Can you work these out from the drawing? Everything is in mm from the part's minimum corner. A direction names the side the tool comes from. Coordinates: 2 decimals unless noted, no trailing zeros. Order: outer loops, then holes, each group sorted by start corner. A loop starts at its lowest first (then second) coordinate and runs counter-clockwise, first axis right, second up. Notation, with made-up numbers: (37.25, -20) -> (68.25, -20) arc R18 cw to (68.25, -5) -> close; hole circle Ø9 at (17.25, 47.25). An arc over 180 degrees is marked (long way). Put each result on its own line as item: value. Start each with the question number.
Q1. Please list where these lines run through material, in increasing order: line 1 along Y through (x, z) = (4.15, 5); line 2 along Z through (x, y) = (2.2, 17.75); line 3 along Z through (x, y) = (0.5, 10).
Q2. If we section it at B-B (x = 3): Please give me the cut outline in (y, z).
Q3. If we section it at A-A (y = 3): Please give me the cut outline in (x, z).
Q4. If we section it at D-D (y = 10.25): Please give me the cut outline in (x, z).
Q5. Will these pins go through, and if not, where does the flat tip stop? pin 1 (3 mm diameter, centred on x = 2, y = 21, fed in from -Z); pin 2 (1.9 mm diameter, centred on x = 3, y = 22.5, fed in from -Z); pin 3 (1 mm diameter, centred on x = 3, y = 12.5, fed in from -Z).
Q6. If we section it at C-C (z = 13.25): Please give me the cut outline in (x, y).
Q7. For the marked faces 1, 2 and 3, which set-ups out of +Z, -Z, +X, -X, +Y, -Y let a thin tool reach every point of the face, with its end or its side?
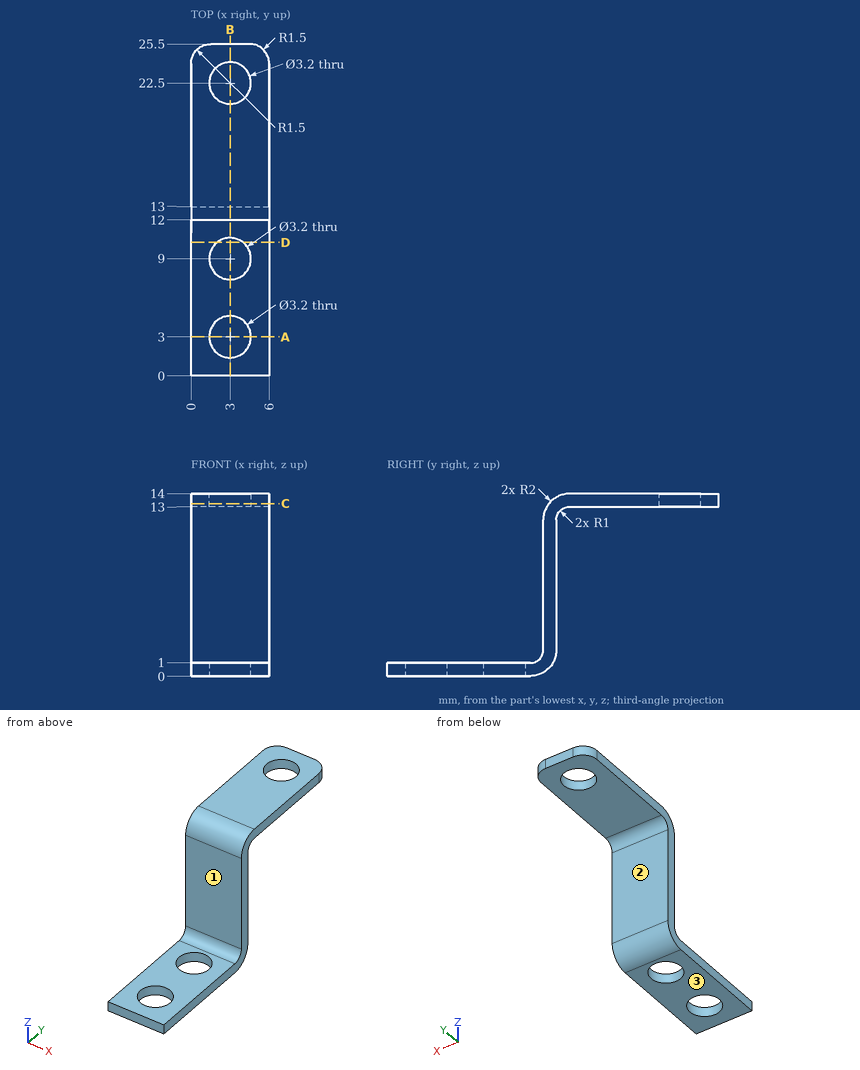
The answers:
1. line 1: 12 to 13
1. line 2: 13 to 14
1. line 3: 0 to 1
2. outline: (0, 0) -> (1.4, 0) -> (1.4, 1) -> (0, 1) -> close; (4.6, 0) -> (7.4, 0) -> (7.4, 1) -> (4.6, 1) -> close; (10.6, 0) -> (11, 0) arc R2 ccw to (13, 2) -> (13, 12) arc R1 cw to (14, 13) -> (20.9, 13) -> (20.9, 14) -> (14, 14) arc R2 ccw to (12, 12) -> (12, 2) arc R1 cw to (11, 1) -> (10.6, 1) -> close; (24.1, 13) -> (25.5, 13) -> (25.5, 14) -> (24.1, 14) -> close
3. outline: (0, 0) -> (1.4, 0) -> (1.4, 1) -> (0, 1) -> close; (4.6, 0) -> (6, 0) -> (6, 1) -> (4.6, 1) -> close
4. outline: (0, 0) -> (2, 0) -> (2, 1) -> (0, 1) -> close; (4, 0) -> (6, 0) -> (6, 1) -> (4, 1) -> close
5. pin 1: z = 13
5. pin 2: through
5. pin 3: z = 0.27
6. outline: (0, 12.44) -> (6, 12.44) -> (6, 24) arc R1.5 ccw to (4.5, 25.5) -> (1.5, 25.5) arc R1.5 ccw to (0, 24) -> close; hole circle Ø3.2 at (3, 22.5)
7. face 1: +Z, +X, -X, -Y
7. face 2: -Z, +X, -X, +Y
7. face 3: -Z, +X, -X, +Y, -Y
